Work out the finished part from the listing and answer in its coordinate system (mm). Coordinates: 2 decimals unless noted, no trailing zeros. Loops run counter-clockwise (first coordinate to the right, second up) from the corner with the lowest first, then second, coordinate; pieces in that order, holes last. Notation, with made-up numbers: (-8, 22.25) -> (26, 22.25) arc R22 cw to (26, 43.25) -> close; hole circle Ø3 at (7.5, -5). An arc over 180 degrees is marked (long way). Use a Markdown table: item, result.
from build123d import *

# Parameters (mm, degrees)
ESBO_O1_W                  = 113
ESBO_O1_H                  = 30
ESBO_O1_R                  = 5
ESBO_O1_R_2                = 3.5
RESSALTO_EXTRUS_O1_DEPTH   = 5.5
ESBO_O2_R                  = 1.5
CORTE_EXTRUS_O1_DEPTH      = 110
CORTE_EXTRUS_O1_DEPTH_BACK = 77.5


with BuildPart() as part:
    # Esboço1 → Ressalto-extrusão1 (new body)
    with BuildSketch(Plane.XY):
        with Locations((-192.217741935, 41.451612903)):
            Rectangle(ESBO_O1_W, ESBO_O1_H)
        with Locations((-192.217741935, 41.451612903)):
            Circle(ESBO_O1_R, mode=Mode.SUBTRACT)
        with Locations((-242.217741935, 41.451612903)):
            Circle(ESBO_O1_R_2, mode=Mode.SUBTRACT)
        with Locations((-142.217741935, 41.451612903)):
            Circle(ESBO_O1_R_2, mode=Mode.SUBTRACT)
    extrude(amount=RESSALTO_EXTRUS_O1_DEPTH)

    # Esboço2 → Corte-extrusão1 (cut, two sides)
    with BuildSketch(Plane(origin=(0, 0, 0), x_dir=(1, 0, 0), z_dir=(0, 1, 0))) as corte_extrus_o1_sk:
        with Locations((-209.217741935, -2.75)):
            Circle(ESBO_O2_R)
        with Locations((-175.217741935, -2.75)):
            Circle(ESBO_O2_R)
    extrude(amount=CORTE_EXTRUS_O1_DEPTH, mode=Mode.SUBTRACT)
    extrude(corte_extrus_o1_sk.sketch, amount=-CORTE_EXTRUS_O1_DEPTH_BACK, mode=Mode.SUBTRACT)


solid = part.part
Q1. Given pin 1 Ø3 at (x, y) = (-170, 31.5) entering from -Z; pin 2 Ø2.5 at (x, z) = (-175.22, 2.75) entering from +Y, each flat-ended and moving along its own axis, determine where each tip first touches the part or whether it passes through.
Solved:
| item | result |
|---|---|
| pin 1 | z = 0 |
| pin 2 | through |
Q2. Section A-A on z = 2.75 is taken. Determine the outline of the cut face in (x, y).
Solved:
| item | result |
|---|---|
| outline | (-248.72, 26.45) -> (-210.72, 26.45) -> (-210.72, 56.45) -> (-248.72, 56.45) -> close; (-207.72, 26.45) -> (-176.72, 26.45) -> (-176.72, 56.45) -> (-207.72, 56.45) -> close; (-173.72, 26.45) -> (-135.72, 26.45) -> (-135.72, 56.45) -> (-173.72, 56.45) -> close; hole circle Ø7 at (-242.22, 41.45); hole circle Ø10 at (-192.22, 41.45); hole circle Ø7 at (-142.22, 41.45) |
Q3. Determine the mould class of faces 1 (the flat face through (-193, 48, 0)), 2 (the flat face through (-193, 56.452, 3)), 3 (the cylindrical face through (-173.83, 41.24, 3.32)) for opening direction Z: pulls with the +Z half, pulls with the -Z half, needs draft (parallel to the pull), parting line crosses it, or undercut.
Solved:
| item | result |
|---|---|
| face 1 | pulls with the -Z half |
| face 2 | needs draft |
| face 3 | undercut |
Q4. Section C-C on y = 28.5 is taken. Determine the outline of the cut face in (x, z).
Solved:
| item | result |
|---|---|
| outline | (-248.72, 0) -> (-135.72, 0) -> (-135.72, 5.5) -> (-248.72, 5.5) -> close; hole circle Ø3 at (-209.22, 2.75); hole circle Ø3 at (-175.22, 2.75) |
Q5. Section B-B on x = -196 is taken. Determine the outline of the cut face in (y, z), and give its area (3 significant figures).
Solved:
| item | result |
|---|---|
| outline | (26.45, 0) -> (38.18, 0) -> (38.18, 5.5) -> (26.45, 5.5) -> close; (44.72, 0) -> (56.45, 0) -> (56.45, 5.5) -> (44.72, 5.5) -> close |
| area | 129 mm² |
Q6. Consider line 1 (X direction, y = 39, z = 3.5); line 2 (X direction, y = 54.5, z = 2.85); line 3 (X direction, y = 55, z = 1.75). Determine where each line is inside the solid, lowest interval first. Write a range as [from, to].
Solved:
| item | result |
|---|---|
| line 1 | [-248.72, -244.72], [-239.72, -210.52], [-207.92, -196.58], [-187.86, -176.52], [-173.92, -144.72], [-139.72, -135.72] |
| line 2 | [-248.72, -210.71], [-207.72, -176.71], [-173.72, -135.72] |
| line 3 | [-248.72, -210.34], [-208.1, -176.34], [-174.1, -135.72] |
